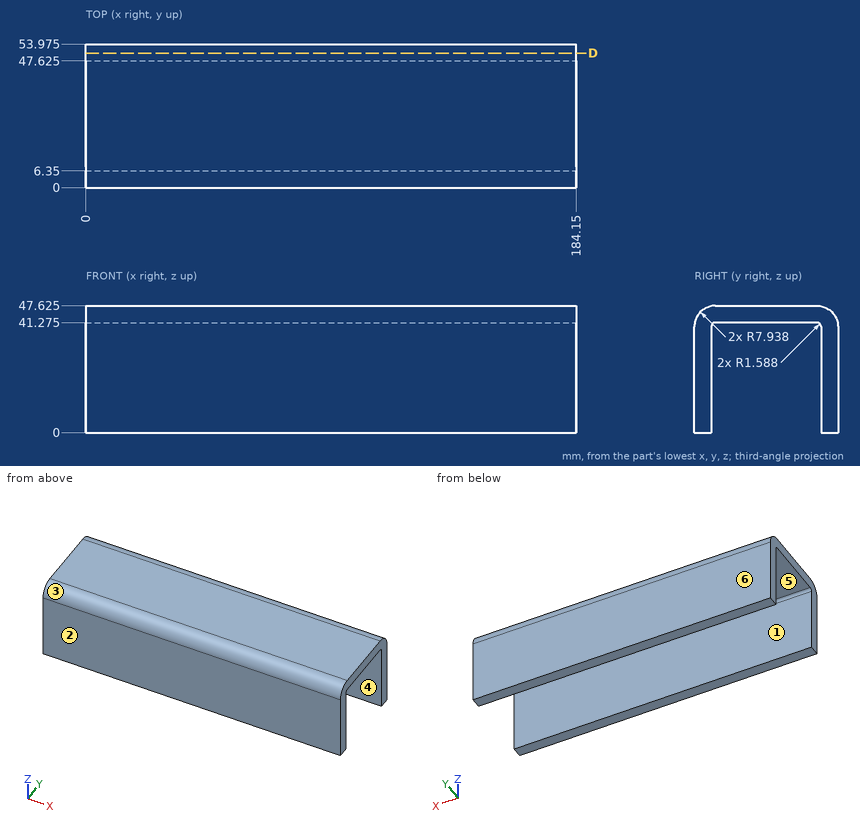
Here's the drawing with two shaded views (mm, measured from the low corner). I have some questions. A direction names the side the tool comes from. Coordinates: 2 decimals unless noted, no trailing zeros. Loops run counter-clockwise (first coordinate to the right, second up) from the corner with the lowest first, then second, coordinate; pieces in that order, holes last.
Item 1: Please list where these lines run through material, in increasing order: L1, parallel to Z at x = 44, y = 9 (1 decimal); L2, parallel to Y at x = 139, z = 44 (1 decimal); L3, parallel to Y at x = 67, z = 43.5 (1 decimal).
Answers below:
L1: z = 41.3 to 47.6
L2: y = 1.3 to 52.7
L3: y = 1 to 53
Item 2: Suppose I cut it at D-D (y = 50.5). Please give me the cut outline in (x, z), then the cut area to 3 significant figures.
Answers below:
outline: (0, 0) - (184.15, 0) - (184.15, 46.25) - (0, 46.25) - close
area: 8,520 mm2
Item 3: If we mould it in two halves opening along Y, with no side actions, what happens to the marked faces 3, 4, 5 and 6? For each: released by +Y, released by -Y, zero draft, split by the parting line, or undercut.
Answers below:
face 3: released by -Y
face 4: undercut
face 5: undercut
face 6: released by +Y
Item 4: Which directions (+Z, -Z, +X, -X, +Y, -Y) give clear straight access to the entire face, cutting with the end or side of a thin tool? Please do the marked faces 1 and 2.
Answers below:
face 1: -Z, +X, -X
face 2: +Z, -Z, +X, -X, -Y
Item 5: I'm going to push flat-ended pins straight in: pin 1 (6 mm diameter, centred on x = 121.5, y = 12, fed in from -Z) (1 decimal); pin 2 (6 mm diameter, centred on y = 42.5, z = 11, fed in from +X); pin 3 (1.5 mm diameter, centred on x = 163, y = 7.5, fed in from -Z). Where does each tip first touch, or does it pass through?
Answers below:
pin 1: stops at z = 41.3
pin 2: passes through
pin 3: stops at z = 40.74
